Here's how the part is built. I have some questions about the finished solid (model axes, mm). A direction names the side the tool comes from. Round coordinates to 2 decimals unless told otherwise and drop trailing zeros. Write each loop counter-clockwise with the first axis right and the second up, starting at its lowest first coordinate (ties: lowest second). Pieces come first, ordered by that corner, then holes. Notation, with made-up numbers: (-29, 9) -> (-14, 9) arc R17 cw to (-14, 22) -> close; hole circle Ø1 at (66.5, 38). An arc over 180 degrees is marked (long way). Put each result on its own line as item: value. Start each with the question number.
1) I want a section at C-C, the plane y = -2.5. List the corners of the cut face in (x, z) for me (1 decimal), then the cut area to 3 significant figures.
2) I want a section at B-B, the plane x = 38. List the corners of the cut face in (y, z) for me, then the cut area to 3 significant figures.
3) Will these pins go through, and if not, where does the flat tip stop? P1, Ø2, axis at y = 3, z = 17.5, coming from the +X side; P2, Ø4, axis at x = -39.5, y = 0.5, coming from the +Z side; P3, Ø1.5, axis at x = -17.5, y = 2, coming from the +Z side.
4) I want a section at A-A, the plane z = 29. List the corners of the cut face in (x, y) for me.
5) We'd pull the mould along X, two halves only. Please class faces 4 (the flat face through (95, 0, 50)), 5 (the cylindrical face through (91, 0, 35)): released by +X, released by -X, zero draft, split by the parting line, or undercut.
6) If I drill on line 1 along X through (y, z) = (-2, 6); line 2 along Z through (x, y) = (-37.5, 0); line 3 along X through (y, z) = (-2.75, 36), over which ranges is the centre line in solid material (lowest first)? Write a range as [from, to].
7) Which directions (+Z, -Z, +X, -X, +Y, -Y) give clear straight access to the entire face, cutting with the end or side of a thin tool? Please do faces 1 (the cylindrical face through (-91, 0, 35)), 2 (the cylindrical face through (-1.05, -0.867, 3.905)), 3 (the flat face through (-95, 0, 50)).
Autodesk Inventor part; units mm, degrees
ref_plane "YZ Plane" through (0, 0, 0) normal (1, 0, 0) x (0, 1, 0)
ref_plane "XZ Plane" through (0, 0, 0) normal (0, 1, 0) x (-1, 0, 0)
ref_plane "XY Plane" through (0, 0, 0) normal (0, 0, 1) x (1, 0, 0)
sketch "Sketch1" plane through (0, 0, 0) normal (1, 0, 0) x (0, 1, 0)
  circle A0 centre (0, 0) radius 4
  dimension "d0" = 8
extrude "Extrusion1" add sketch "Sketch1" along normal mid plane 150
sketch "Sketch4" plane through (75, 0, 0) normal (1, 0, 0) x (0, 0, -1)
  circle A0 centre (0, 0) radius 4
  line L0 (-20, 15.4363) -> (-20, -7.2727)
  circle A1 centre (0, 0) radius 4
  dimension "d10" = 20
  dimension "d11" = 0
revolve "Revolution1" add sketch "Sketch4" angle 90 about axis through (75, 15.4363, 20) along (0, -1, 0)
mirror "Mirror1" about plane through (0, 0, 0) normal (1, 0, 0) of "Revolution1"
sketch "Sketch5" plane through (95, 0, 20) normal (0, 0, 1) x (1, 0, 0)
  circle A0 centre (0, 0) radius 4
  point P0 (-95, 0)
extrude "Extrusion3" add sketch "Sketch5" along normal blind 30
mirror "Mirror2" about plane through (0, 0, 0) normal (1, 0, 0) of "Extrusion3"
sketch "Sketch6" plane through (95, 0, 50) normal (0, 0, 1) x (1, 0, 0)
  circle A0 centre (0, 0) radius 4
  line L0 (-1.147, 3.832) -> (3.8236, 3.832)
  line L1 (3.8236, 3.832) -> (3.8236, -1.1749)
  line L2 (3.8236, -1.1749) -> (-1.147, -1.1749)
  line L3 (-1.147, -1.1749) -> (-1.147, 3.832)
  circle A1 centre (0, 0) radius 4
  point P0 (-95, 0)
  point P1 (3.8236, 1.1749)
  point P2 (1.147, 3.832)
extrude "Extrusion4" cut sketch "Sketch6" against normal blind 1 contours A0 L0 | L1 A0
properties part number "Handle"
Findings:
1. outline: (-98.1, 20) arc R23.1 ccw to (-75, -3.1) -> (75, -3.1) arc R23.1 ccw to (98.1, 20) -> (98.1, 50) -> (91.9, 50) -> (91.9, 20) arc R16.9 cw to (75, 3.1) -> (-75, 3.1) arc R16.9 cw to (-91.9, 20) -> (-91.9, 50) -> (-98.1, 50) -> close
1. area: 1,700 mm2
2. outline: circle Ø8 at (0, 0)
2. area: 50.3 mm2
3. P1: stops at x = 98.34
3. P2: stops at z = 4
3. P3: stops at z = 3.8
4. outline: circle Ø8 at (-95, 0); circle Ø8 at (95, 0)
5. face 4: zero draft
5. face 5: undercut
6. line 1: x = [-93.83, -83.8], [83.8, 93.83]
6. line 2: z = [-4, 4]
6. line 3: x = [-97.9, -92.1], [92.1, 97.9]
7. face 1: +Z
7. face 2: none
7. face 3: +Z, +X, -X, +Y, -Y
